Read the model definition and answer for the solid it produces. Units are mm, in the model's axes. Face numbers are marked on the shaded views. A direction names the side the tool comes from. Give positions to 0.01 mm unless a question says otherwise; leave off trailing zeros. Order: outer loops, then holes, each group sorted by start corner. A loop starts at its lowest first (then second) coordinate and runs counter-clockwise, first axis right, second up. Notation, with made-up numbers: (-31.5, 18) - (12.5, 18) arc R25 ccw to (12.5, 42) - close; hole circle Ø10 at (-26.5, 59). An arc over 180 degrees is marked (long way). Return JSON: item names as keys, results as strings.
Autodesk Inventor part; units mm, degrees
ref_plane "YZ Plane" through (0, 0, 0) normal (1, 0, 0) x (0, 1, 0)
ref_plane "XZ Plane" through (0, 0, 0) normal (0, 1, 0) x (-1, 0, 0)
ref_plane "XY Plane" through (0, 0, 0) normal (0, 0, 1) x (1, 0, 0)
sketch "Sketch1" plane through (0, 0, 0) normal (0, 1, 0) x (-1, 0, 0)
  line L0 (0, 0) -> (25.4, 0)
  line L1 (25.4, 0) -> (25.4, 25.4)
  line L2 (25.4, 25.4) -> (0, 25.4)
  line L3 (0, 25.4) -> (0, 0)
  line L4 (3.175, 22.225) -> (22.225, 22.225)
  line L5 (22.225, 22.225) -> (22.225, 3.175)
  line L6 (22.225, 3.175) -> (3.175, 3.175)
  line L7 (3.175, 3.175) -> (3.175, 22.225)
  dimension "d0" = 25.4
  dimension "d1" = 25.4
  dimension "d2" = 3.175
extrude "Extrusion1" add sketch "Sketch1" along normal blind 19.05
sketch "Sketch2" plane through (-25.4, 0, 25.4) normal (0, 0, 1) x (1, 0, 0)
  line L0 (0, 0) -> (25.4, 0)
  line L1 (25.4, 0) -> (25.4, 19.05)
  line L2 (0, 19.05) -> (25.4, 19.05)
  line L3 (0, 0) -> (0, 19.05)
  line L4 (0, 9.525) -> (25.4, 9.525) construction
  line L5 (12.7, 19.05) -> (12.7, 0) construction
  circle A0 centre (12.7, 9.525) radius 3.302
  dimension "d5" = 6.604
extrude "Extrusion2" cut sketch "Sketch2" against normal blind 25.4 contours A0
sketch "Sketch3" plane through (0, 0, 0) normal (0, 0, -1) x (-1, 0, 0)
  circle A0 centre (12.7, 9.525) radius 3.302
  circle A1 centre (12.7, 9.525) radius 6.35
  dimension "d9" = 12.7
extrude "Extrusion3" cut sketch "Sketch3" against normal blind 3.175
properties part number "Chassis Part 12 (26x28)" material "Aluminum 6061"
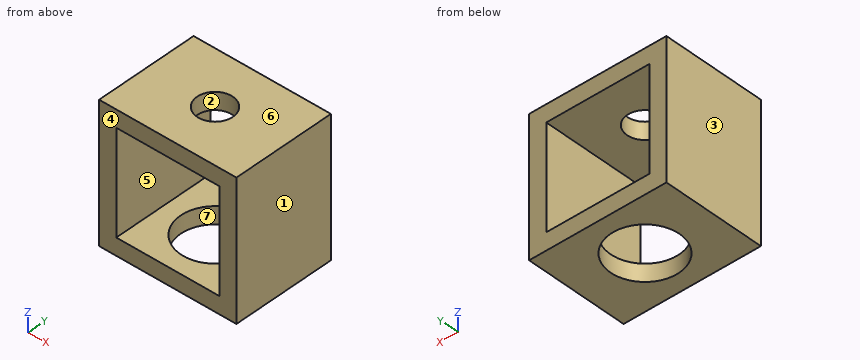
Q1. Consider L1, parallel to X at y = 3.75, z = 16 (3 decimals); L2, parallel to Y at x = -12.7, z = 23; L3, parallel to Z at x = -5, y = 11 (3 decimals). Determine where each line is inside the solid, lowest interval first.
Values:
{"L1": "x = -25.4 to -22.225, -3.175 to 0", "L2": "y = 0 to 6.22, 12.83 to 19.05", "L3": "z = 0 to 3.175, 22.225 to 25.4"}
Q2. A cutting plane is placed at C-C (z = 4). Write down the section's boundary in (x, y) (3 decimals).
Values:
{"outline": "(-25.4, 0) - (-22.225, 0) - (-22.225, 19.05) - (-25.4, 19.05) - close; (-3.175, 0) - (0, 0) - (0, 19.05) - (-3.175, 19.05) - close"}
Q3. A cutting plane is placed at D-D (y = 2.75). Write down the section's boundary in (x, z) (3 decimals), and give its area (3 significant figures).
Values:
{"outline": "(-25.4, 0) - (0, 0) - (0, 25.4) - (-25.4, 25.4) - close; hole (-22.225, 3.175) - (-3.175, 3.175) - (-3.175, 22.225) - (-22.225, 22.225) - close", "area": "282 mm²"}
Q4. A cutting plane is placed at A-A (x = -5). Write down the section's boundary in (y, z) (3 decimals), and give its area (3 significant figures).
Values:
{"outline": "(0, 0) - (19.05, 0) - (19.05, 3.175) - (0, 3.175) - close; (0, 22.225) - (19.05, 22.225) - (19.05, 25.4) - (0, 25.4) - close", "area": "121 mm²"}
Q5. For the marked faces 5, 6 and 7, determine the directions among +Z, -Z, +X, -X, +Y, -Y from which every point of the face is accessible in a straight line to the end or side of a thin tool.
Values:
{"face 5": "+Y, -Y", "face 6": "+Z, +X, -X, +Y, -Y", "face 7": "-Z"}
Q6. Determine the mould class of the marked faces 1, 2, 3 and 4 for opening direction X: released by +X, released by -X, zero draft, split by the parting line, or undercut.
Values:
{"face 1": "released by +X", "face 2": "undercut", "face 3": "released by -X", "face 4": "zero draft"}
Q7. A cutting plane is placed at B-B (x = -12.7). Write down the section's boundary in (y, z) (3 decimals), and give its area (3 significant figures).
Values:
{"outline": "(0, 0) - (3.175, 0) - (3.175, 3.175) - (0, 3.175) - close; (0, 22.225) - (6.223, 22.225) - (6.223, 25.4) - (0, 25.4) - close; (12.827, 22.225) - (19.05, 22.225) - (19.05, 25.4) - (12.827, 25.4) - close; (15.875, 0) - (19.05, 0) - (19.05, 3.175) - (15.875, 3.175) - close", "area": "59.7 mm²"}
